Read the model definition and answer for the solid it produces. Units are mm, in the model's axes. A direction names the side the tool comes from. Give positions to 0.01 mm unless a question says otherwise; leave off trailing zeros. Loops run counter-clockwise (first coordinate to the right, second up) from the corner with the lowest first, then second, coordinate; pieces in that order, holes last. Notation, with made-up numbers: (-18.75, 64.5) - (5.25, 64.5) arc R34 cw to (5.25, 95.5) - close; hole circle Ø6 at (-21.75, 19). An arc over 180 degrees is marked (long way). Write each question's results on one line, items separated by ' | '. Start each with the question number.
Q1. For faces 4 (the flat face through (25, 3, 1)), 5 (the flat face through (24, 13.5, 1)), 6 (the flat face through (2, 10, 1)), determine the directions among +Z, -Z, +X, -X, +Y, -Y from which every point of the face is accessible in a straight line to the end or side of a thin tool.
Q2. Determine the mould class of faces 1 (the flat face through (13, 12, 0)), 2 (the flat face through (23, 10, 1)), 3 (the flat face through (13, 0, 1)) for opening direction Y: +Y half, -Y half, draft (parallel to the pull), parting line (faces both ways), or undercut.
Q3. Find the intervals of material crossed by line 1 (Y direction, x = 1, z = 0.6); line 2 (X direction, y = 9, z = 1.25); line 3 (X direction, y = 15, z = 2.9), in increasing order. Write a range as from..to.
Q4. Given pin 1 (1.5 mm diameter, centred on y = 9.5, z = 1.5, fed in from +X), flat-ended and moving along its own axis, determine where the tip first touches the part or whether it passes through.
Q5. The part is cut by section B-B, the plane y = 12. Write down the section's boundary in (x, z).
Q6. The part is cut by section A-A, the plane z = 0.6. Write down the section's boundary in (x, y), plus the area to 3 significant figures.
```python
from build123d import *

# Parameters (mm, degrees)
EXTRUDE_1_DEPTH = 3
CHAMFER_1_SIZE  = 0.25


with BuildPart() as part:
    # Эскиз1 → Бобышка-Вытянуть1 (new body)
    with BuildSketch(Plane.XY):
        with BuildLine():
            Line((0, 0), (0, 6.5))
            Line((0, 6.5), (1.7, 6.5))
            ThreePointArc((1.7, 6.5), (1.912132034, 6.587867966), (2, 6.8))
            Line((2, 6.8), (2, 13.2))
            ThreePointArc((2, 13.2), (1.912132034, 13.412132034), (1.7, 13.5))
            Line((1.7, 13.5), (0, 13.5))
            Line((0, 13.5), (0, 23.5))
            Line((0, 23.5), (25, 23.5))
            Line((25, 23.5), (25, 13.5))
            Line((25, 13.5), (23.3, 13.5))
            ThreePointArc((23.3, 13.5), (23.087867966, 13.412132034), (23, 13.2))
            Line((23, 13.2), (23, 6.8))
            ThreePointArc((23, 6.8), (23.087867966, 6.587867966), (23.3, 6.5))
            Line((23.3, 6.5), (25, 6.5))
            Line((25, 6.5), (25, 0))
            Line((25, 0), (0, 0))
        make_face()
    extrude(amount=EXTRUDE_1_DEPTH)

    # Фаска1
    chamfer_1_edges = [part.edges().sort_by_distance(p)[0] for p in [
        (25, 18.5, 3),
        (12.5, 23.5, 3),
        (0, 18.5, 3),
    ]]
    chamfer(chamfer_1_edges, length=CHAMFER_1_SIZE)


solid = part.part
```
Check sheet entries:
1) face 4: +Z, -Z, +X, +Y, -Y | face 5: +Z, -Z, +X | face 6: +Z, -Z, -X
2) face 1: draft | face 2: undercut | face 3: -Y half
3) line 1: y = 0..6.5, 13.5..23.5 | line 2: x = 2..23 | line 3: x = 0.15..24.85
4) pin 1: stops at x = 23
5) outline: (2, 0) - (23, 0) - (23, 3) - (2, 3) - close
6) outline: (0, 0) - (25, 0) - (25, 6.5) - (23.3, 6.5) arc R0.3 cw to (23, 6.8) - (23, 13.2) arc R0.3 cw to (23.3, 13.5) - (25, 13.5) - (25, 23.5) - (0, 23.5) - (0, 13.5) - (1.7, 13.5) arc R0.3 cw to (2, 13.2) - (2, 6.8) arc R0.3 cw to (1.7, 6.5) - (0, 6.5) - close | area: 560 mm^2
